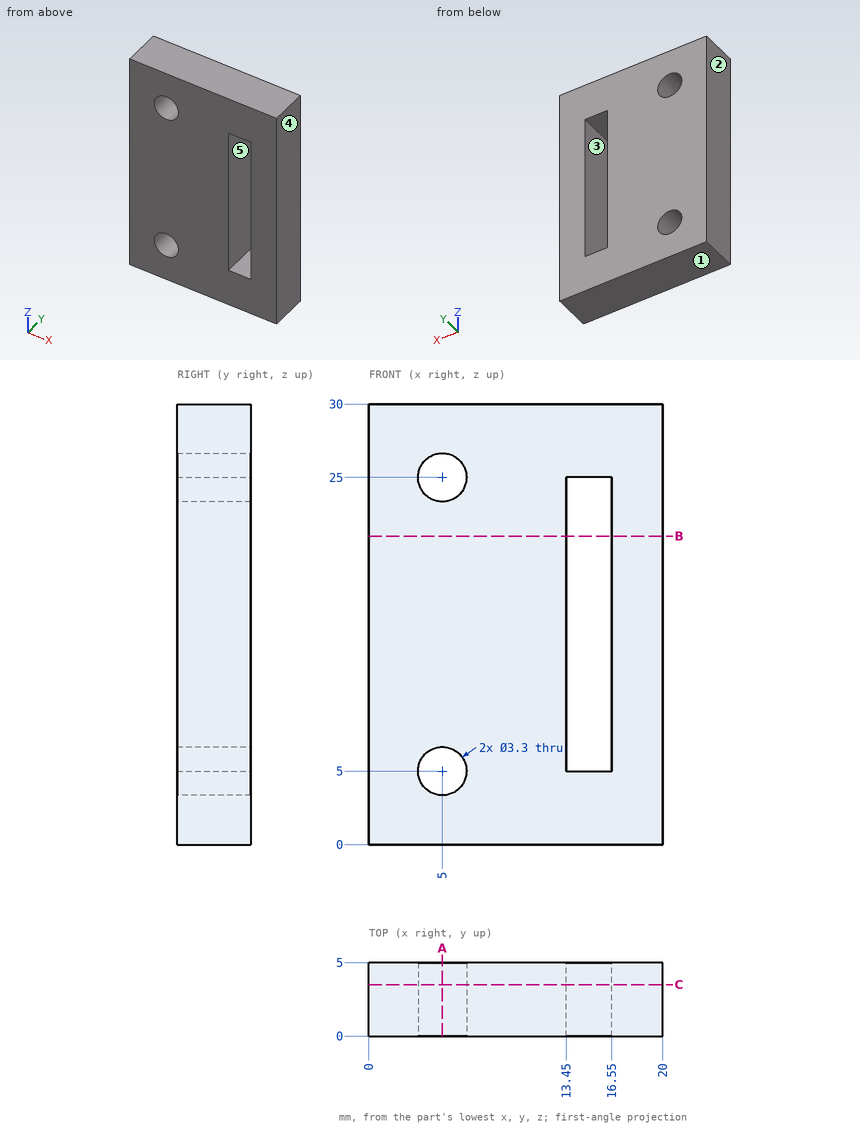
Check sheet for the drawn part. Datum: minimum x, y, z corner. Units: mm. A direction names the side the tool comes from. Round coordinates to 2 decimals unless told otherwise and drop trailing zeros. Write each loop counter-clockwise with the first axis right and the second up, starting at its lowest first coordinate (ties: lowest second). Pieces come first, ordered by that corner, then holes. Notation, with made-up numbers: (14, 45) - (66, 45) arc R28 ccw to (66, 70) - close; hole circle Ø3 at (12.5, 57.5). An arc over 180 degrees is marked (long way). Return JSON: item names as keys, results as strings.
Q1. Access from +Z, -Z, +X, -X, +Y, -Y to the whole of each face (thin tool, end or side, straight path). Record for the marked faces 4 and 5.
Returned:
{"face 4": "+Z, -Z, +X, +Y, -Y", "face 5": "+Y, -Y"}
Q2. Scan lines: L1, parallel to Z at x = 15.25, y = 0.6; L2, parallel to X at y = 1.5, z = 8.5; L3, parallel to Z at x = 5.5, y = 2.1. Record each from-to range of solid material in increasing order. Write a range as from..to.
Returned:
{"L1": "z = 0..5, 25..30", "L2": "x = 0..13.45, 16.55..20", "L3": "z = 0..3.43, 6.57..23.43, 26.57..30"}
Q3. Cross-section at B-B (z = 21). Record the boundary of the cut face in (x, y), then the cut area to 3 significant figures.
Returned:
{"outline": "(0, 0) - (13.45, 0) - (13.45, 5) - (0, 5) - close; (16.55, 0) - (20, 0) - (20, 5) - (16.55, 5) - close", "area": "84.5 mm²"}
Q4. Depth check by flat-ended pin: P1, Ø1.5, axis at x = 6, z = 16.5, coming from the -Y side. Enter the tip coordinate at first touch or a pass-through.
Returned:
{"P1": "stops at y = 0"}
Q5. Draft check along Z on the marked faces 1, 2 and 3. Enter one of: released by +Z, released by -Z, zero draft, split by the parting line, or undercut.
Returned:
{"face 1": "released by -Z", "face 2": "zero draft", "face 3": "undercut"}
Q6. Cross-section at C-C (y = 3.5). Record the boundary of the cut face in (x, z), then the cut area to 3 significant figures.
Returned:
{"outline": "(0, 0) - (20, 0) - (20, 30) - (0, 30) - close; hole circle Ø3.3 at (5, 5); hole circle Ø3.3 at (5, 25); hole (13.45, 5) - (16.55, 5) - (16.55, 25) - (13.45, 25) - close", "area": "521 mm²"}
Q7. Cross-section at A-A (x = 5). Record the boundary of the cut face in (y, z).
Returned:
{"outline": "(0, 0) - (5, 0) - (5, 3.35) - (0, 3.35) - close; (0, 6.65) - (5, 6.65) - (5, 23.35) - (0, 23.35) - close; (0, 26.65) - (5, 26.65) - (5, 30) - (0, 30) - close"}
